Source: CAD feature listing. Evaluate the final solid. Frame: model axes, mm. A direction names the side the tool comes from. Coordinates: 2 decimals unless noted, no trailing zeros. Write each loop counter-clockwise with the first axis right and the second up, starting at its lowest first coordinate (ties: lowest second). Pieces come first, ordered by that corner, then holes. Notation, with made-up numbers: M 15.25,38 L 42.25,38 A15 ccw 42.25,54 Z; hole C -5.5,-32.75 d8. An arc over 180 degrees is marked long. Answer as CSV lines item,"result". Start each with the question number.
1. Reachability of faces 1 (the face through (0, -55, 5)), 2 (the face through (-0.751, -32.185, 7.385)), 3 (the face through (-1.2, -1.2, 2.5)) from +Z, -Z, +X, -X, +Y, -Y: full face, straight path, thin tool, end or side. Return the list, or none.
2. Contact query for flat-ended pins moving along their axis: pin 1 Ø4 at (x, y) = (3, -36.5) entering from -Z; pin 2 Ø5.5 at (x, z) = (-2.5, 4.5) entering from +Y; pin 3 Ø6 at (y, z) = (-28, 6) entering from +X. Output: stop coordinate, or through.
3. Line query: probe 1 along Y at (x, z) = (0, 9.3); probe 2 along Z at (x, y) = (1.5, -1); probe 3 along X at (y, z) = (-18.5, 7). Output: solid intervals per line, ascending. Write a range as [from, to].
4. Section A-A on x = 0. Return the cut outline in (y, z), plus the area to 3 significant figures.
5. Section C-C on z = 5. Return the cut outline in (x, y), plus the area to 3 significant figures.
6. Section B-B on z = 1.5. Return the cut outline in (x, y).
7. Section D-D on y = -37. Return the cut outline in (x, z), plus the area to 3 significant figures.
8. Mould query, pull axis Z, two halves, no side actions, for faces 4 (the face through (0, 5, 9)), 5 (the face through (0, -2, 0)), 6 (the face through (0, -5, 5)). Classes: pulls with the +Z half, pulls with the -Z half, needs draft (parallel to the pull), parting line crosses it, or undercut.
```python
from build123d import *

# Parameters (mm, degrees)
CROQUIS1_R              = 1.5
SALIENTE_EXTRUIR1_DEPTH = 10
CROQUIS2_R              = 2.5
SALIENTE_EXTRUIR2_DEPTH = 45
CROQUIS3_W              = 5
CROQUIS3_H              = 10
CORTAR_EXTRUIR1_DEPTH   = 40


with BuildPart() as part:
    # Croquis1 → Saliente-Extruir1 (new body)
    with BuildSketch(Plane.XY):
        with BuildLine():
            Line((-5, 0), (-5, -10))
            Line((-5, -10), (5, -10))
            Line((5, -10), (5, 0))
            ThreePointArc((5, 0), (0, 5), (-5, 0))
        make_face()
        Circle(CROQUIS1_R, mode=Mode.SUBTRACT)
    extrude(amount=SALIENTE_EXTRUIR1_DEPTH)

    # Croquis2 → Saliente-Extruir2 (add)
    with BuildSketch(Plane.XZ.offset(10)):
        with Locations(Location((0, 5, 0), (0, 0, 90))):
            Circle(CROQUIS2_R)
    extrude(amount=SALIENTE_EXTRUIR2_DEPTH)

    # Croquis3 → Cortar-Extruir1 (cut)
    with BuildSketch(Plane.ZY.offset(5)):
        with Locations((5, 0)):
            Rectangle(CROQUIS3_W, CROQUIS3_H)
    extrude(amount=-CORTAR_EXTRUIR1_DEPTH, mode=Mode.SUBTRACT)


solid = part.part
```
Values:
1,face 1,"+Z, -Z, +X, -X, -Y"
1,face 2,"-Y"
1,face 3,"+X, -X, +Y"
2,pin 1,"z = 2.71"
2,pin 2,"y = 4.96"
2,pin 3,"x = 2.5"
3,probe 1,"[-10, -1.5], [1.5, 5]"
3,probe 2,"[0, 2.5], [7.5, 10]"
3,probe 3,"[-1.5, 1.5]"
4,outline,"M -55,2.5 L -10,2.5 L -10,0 L -1.5,0 L -1.5,2.5 L -5,2.5 L -5,7.5 L -1.5,7.5 L -1.5,10 L -10,10 L -10,7.5 L -55,7.5 Z; M 1.5,0 L 5,0 L 5,2.5 L 1.5,2.5 Z; M 1.5,7.5 L 5,7.5 L 5,10 L 1.5,10 Z"
4,area,"310 mm²"
5,outline,"M -5,-10 L -2.5,-10 L -2.5,-55 L 2.5,-55 L 2.5,-10 L 5,-10 L 5,-5 L -5,-5 Z"
5,area,"275 mm²"
6,outline,"M -5,-10 L 5,-10 L 5,0 A5 ccw -5,0 Z; hole C 0,0 d3"
7,outline,"C 0,5 d5"
7,area,"19.6 mm²"
8,face 4,"needs draft"
8,face 5,"pulls with the -Z half"
8,face 6,"undercut"
